from build123d import *

# Parameters (mm, degrees)
F0_W     = 304.8
F0_H     = 406.4
F0_R     = 11.1125
F1_DEPTH = 1.651
F2_W     = 304.8
F2_H     = 406.4
F2_W_2   = 301.498
F2_H_2   = 403.098
F3_DEPTH = 19.05
F4_R     = 5.08
F5_R     = 5.08
F6_R     = 2.54
F7_DEPTH = 25.4


with BuildPart() as f1:
    # F0 (on Front) → F1 (new body)
    with BuildSketch(Plane.XZ):
        Rectangle(F0_W, F0_H)
        with BuildLine():
            Line((-127, 177.8), (127, 177.8))
            Line((127, 177.8), (127, 76.651281))
            Line((127, 76.651281), (72.79936, 22.45064))
            ThreePointArc((72.79936, 22.45064), (63.5, 0), (72.79936, -22.45064))
            Line((72.79936, -22.45064), (127, -76.651281))
            Line((127, -76.651281), (127, -177.8))
            Line((127, -177.8), (-127, -177.8))
            Line((-127, -177.8), (-127, 177.8))
        make_face(mode=Mode.SUBTRACT)
        with Locations((95.25, 0)):
            Circle(F0_R, mode=Mode.SUBTRACT)
    extrude(amount=F1_DEPTH)

    # F2 (on face) → F3 (join)
    with BuildSketch(Plane.XZ.offset(1.651)):
        Rectangle(F2_W, F2_H)
        Rectangle(F2_W_2, F2_H_2, mode=Mode.SUBTRACT)
    extrude(amount=-F3_DEPTH)

    # F4
    f4_edges = [f1.edges().sort_by_distance(p)[0] for p in [
        (-150.749, 0, 0),
        (0, 0, 201.549),
        (150.749, 0, 0),
        (0, 0, -201.549),
        (-150.749, 8.6995, -201.549),
        (-150.749, 8.6995, 201.549),
        (150.749, 8.6995, 201.549),
        (150.749, 8.6995, -201.549),
    ]]
    fillet(f4_edges, radius=F4_R)

    # F5
    f5_edges = [f1.edges().sort_by_distance(p)[0] for p in [
        (-152.4, 7.874, 203.2),
        (0, -1.651, 203.2),
        (-152.4, -1.651, 0),
        (152.4, 7.874, 203.2),
        (152.4, -1.651, 0),
        (152.4, 7.874, -203.2),
        (0, -1.651, -203.2),
        (-152.4, 7.874, -203.2),
    ]]
    fillet(f5_edges, radius=F5_R)

    # F6 (on face) → F7 (cut)
    with BuildSketch(Plane.XZ.offset(1.651)):
        with Locations((-133.35, 184.15)):
            Circle(F6_R)
        with Locations((-133.35, 92.075)):
            Circle(F6_R)
        with Locations((-133.35, 0)):
            Circle(F6_R)
        with Locations((-133.35, -92.075)):
            Circle(F6_R)
        with Locations((-133.35, -184.15)):
            Circle(F6_R)
        with Locations((-44.45, 184.15)):
            Circle(F6_R)
        with Locations((44.45, 184.15)):
            Circle(F6_R)
        with Locations((133.35, 184.15)):
            Circle(F6_R)
        with Locations((133.35, 92.075)):
            Circle(F6_R)
        with Locations((133.35, -92.075)):
            Circle(F6_R)
        with Locations((133.35, -184.15)):
            Circle(F6_R)
        with Locations((44.45, -184.15)):
            Circle(F6_R)
        with Locations((-44.45, -184.15)):
            Circle(F6_R)
        with Locations((69.85, 0)):
            Circle(F6_R)
    extrude(amount=-F7_DEPTH, mode=Mode.SUBTRACT)


solid = f1.part
Model file for the job. Use its own axes, mm. A direction names the side the tool comes from. Coordinates: 2 decimals unless noted, no trailing zeros. Order: outer loops, then holes, each group sorted by start corner. A loop starts at its lowest first (then second) coordinate and runs counter-clockwise, first axis right, second up. Notation, with made-up numbers: (-39.75, 22) -> (-34.75, 22) arc R25 ccw to (-34.75, 43) -> close; hole circle Ø9 at (35, 39). An arc over 180 degrees is marked (long way). Return JSON: item names as keys, results as strings. Group by question number.
Item 1: Wall check: line 1 along Z through (x, y) = (-133.35, -0.35) (3 decimals); line 2 along X through (y, z) = (6.25, -0.5); line 3 along Z through (x, y) = (-44.45, -1.2). Give the ranges that are in metal, low to high. Write a range as [from, to].
Item 2: Saw through at D-D on x = 93.5. Write the cut outline in (y, z), then the cut area to 3 significant figures.
Item 3: Tool access for faces 5 (the flat face through (150.749, 11, -3)), 6 (the cylindrical face through (63.5, -0.8, 0.3)), 7 (the flat face through (65, -1.651, 1)): list every direction of +Z, -Z, +X, -X, +Y, -Y with a clear straight run to the whole face (end or side of a thin tool).
Item 4: Saw through at A-A on x = -67.5. Write the cut outline in (y, z).
Item 5: Flat gauge pins, fed straight in: P1, Ø0.8, axis at y = -1, z = -146.5, coming from the -X side; P2, Ø0.8, axis at x = -63.5, y = -0.5, coming from the -Z side; P3, Ø8, axis at x = 133.35, z = -184.15, coming from the +Y side. Where does each tip first touch, or does it go through?
Item 6: Saw through at B-B on y = 9.5. Write the cut outline in (x, z).
Item 7: Pull direction X, two halves, no side cores. Call faces 1 (the flat face through (152.4, 10, -3)), 2 (the flat face through (99.52, -0.81, -49.17)), 3 (the flat face through (-2, 10, 203.2)), 4 (the cylindrical face through (84.15, -0.81, 0.49)): pulls with the +X half, pulls with the -X half, needs draft (parallel to the pull), parting line crosses it, or undercut.
Item 8: Saw through at C-C on z = -159. Write the cut outline in (x, y).
Values found:
{
 "1": {"line 1": "z = [-201.515, -186.69], [-181.61, -94.615], [-89.535, -2.54], [2.54, 89.535], [94.615, 181.61], [186.69, 201.515]", "line 2": "x = [-152.4, -150.75], [150.75, 152.4]", "line 3": "z = [-200.21, -186.69], [-181.61, -177.8], [177.8, 181.61], [186.69, 200.21]"},
 "2": {"outline": "(-1.65, -198.12) arc R5.08 ccw to (3.43, -203.2) -> (17.4, -203.2) -> (17.4, -201.55) -> (5.08, -201.55) arc R5.08 cw to (0, -196.47) -> (0, -177.8) -> (-1.65, -177.8) -> close; (-1.65, -43.15) -> (0, -43.15) -> (0, -10.97) -> (-1.65, -10.97) -> close; (-1.65, 10.97) -> (0, 10.97) -> (0, 43.15) -> (-1.65, 43.15) -> close; (-1.65, 177.8) -> (0, 177.8) -> (0, 196.47) arc R5.08 cw to (5.08, 201.55) -> (17.4, 201.55) -> (17.4, 203.2) -> (3.43, 203.2) arc R5.08 ccw to (-1.65, 198.12) -> close", "area": "248 mm2"},
 "3": {"face 5": "+Y", "face 6": "+Y, -Y", "face 7": "+Z, -Z, +X, -X, -Y"},
 "4": {"outline": "(-1.65, -198.12) arc R5.08 ccw to (3.43, -203.2) -> (17.4, -203.2) -> (17.4, -201.55) -> (5.08, -201.55) arc R5.08 cw to (0, -196.47) -> (0, -177.8) -> (-1.65, -177.8) -> close; (-1.65, 177.8) -> (0, 177.8) -> (0, 196.47) arc R5.08 cw to (5.08, 201.55) -> (17.4, 201.55) -> (17.4, 203.2) -> (3.43, 203.2) arc R5.08 ccw to (-1.65, 198.12) -> close"},
 "5": {"P1": "stops at x = -150.41", "P2": "stops at z = -201.77", "P3": "stops at y = 0"},
 "6": {"outline": "(-152.4, -198.12) arc R5.08 ccw to (-147.32, -203.2) -> (147.32, -203.2) arc R5.08 ccw to (152.4, -198.12) -> (152.4, 198.12) arc R5.08 ccw to (147.32, 203.2) -> (-147.32, 203.2) arc R5.08 ccw to (-152.4, 198.12) -> close; hole (-150.75, -196.47) arc R5.08 ccw to (-145.67, -201.55) -> (145.67, -201.55) arc R5.08 ccw to (150.75, -196.47) -> (150.75, 196.47) arc R5.08 ccw to (145.67, 201.55) -> (-145.67, 201.55) arc R5.08 ccw to (-150.75, 196.47) -> close"},
 "7": {"face 1": "pulls with the +X half", "face 2": "undercut", "face 3": "needs draft", "face 4": "undercut"},
 "8": {"outline": "(-152.4, 3.43) arc R5.08 ccw to (-147.32, -1.65) -> (-127, -1.65) -> (-127, 0) -> (-145.67, 0) arc R5.08 cw to (-150.75, 5.08) -> (-150.75, 17.4) -> (-152.4, 17.4) -> close; (127, -1.65) -> (147.32, -1.65) arc R5.08 ccw to (152.4, 3.43) -> (152.4, 17.4) -> (150.75, 17.4) -> (150.75, 5.08) arc R5.08 cw to (145.67, 0) -> (127, 0) -> close"}
}
